Solid Edge part; units mm, degrees
sketch "Sketch1" plane through (0, 0, 0) normal (1, 0, 0) x (0, 1, 0)
  line L0 (-22.5, 0) -> (22.5, 0)
  line L1 (22.5, 0) -> (22.5, 6)
  line L2 (22.5, 6) -> (13.5, 6)
  line L3 (13.5, 6) -> (11, 21)
  arc A0 (-11, 21) -> (11, 21) centre (0, 21) cw
  line L4 (-13.5, 6) -> (-11, 21)
  line L5 (-22.5, 6) -> (-13.5, 6)
  line L6 (-22.5, 0) -> (-22.5, 6)
  dimension "D1" = 22.5
  dimension "D2" = 22.5
  dimension "D3" = 22.5
extrude "Protrusion1" add sketch "Sketch1" along normal mid plane 8
hole "Hole_1" at (0, -18, 6) direction (0, 0, -1) diameter 4.5 end up to next start chamfer 0.4 start chamfer angle 30
hole "Hole1" at (0, 18, 6) direction (0, 0, -1) diameter 4.5 end up to next start chamfer 0.4 start chamfer angle 30
chamfer "Chamfer_1" distance 2 angle 45 4 edges at (4, -22.5, 3) (-4, -22.5, 3) (-4, 22.5, 3) (4, 22.5, 3)
hole "Hole_3" at (4, 0, 21) direction (-1, 0, 0) diameter 12.6 end up to next start chamfer 1 start chamfer angle 30 end chamfer 1 end chamfer angle 30
properties material "Polyethylene, low density"
The model under review builds one solid part; all positions refer to its coordinate system, in mm. A direction names the side the tool comes from. Round coordinates to 2 decimals unless told otherwise and drop trailing zeros. Order: outer loops, then holes, each group sorted by start corner. A loop starts at its lowest first (then second) coordinate and runs counter-clockwise, first axis right, second up. Notation, with made-up numbers: (30, 13) -> (47, 13) arc R4 ccw to (47, 18) -> close; hole circle Ø11 at (13.5, 49.5). An arc over 180 degrees is marked (long way). One line per item, written item: value. Start each with the question number.
Q1. Take a section at B-B (y = -18). Write out the cut boundary in (x, z).
Q2. Take a section at D-D (x = 1). Count the separate pieces of the cut face and the enclosed holes in it, and give its area (3 significant figures).
Q3. Wall thickness on line 1 (Y direction, x = 0, z = 1.1); line 2 (X direction, y = -18, z = 1); line 3 (Y direction, x = 0.05, z = 21): over which ranges is each line inside the solid? List them lowest first.
Q4. Machinability: for faces 5 (the face through (-2, -16, 6)), 6 (the face through (0, 0, 0)), which of the approach directions +Z, -Z, +X, -X, +Y, -Y give a long, thin tool a straight path to every point of the face, cutting with its end or side? Answer none if there is none.
Q5. Clearance check with flat-ended pins moving along their axes: pin 1 Ø1 at (x, y) = (3, -2) entering from +Z; pin 2 Ø4 at (x, z) = (2.5, 17) entering from -Y; pin 3 Ø3 at (x, z) = (-3, 16.5) entering from +Y. State where each tip first meets the part, or that it passes through.
Q6. Take a section at A-A (z = 4). Write out the cut boundary in (x, y).
Q7. Take a section at C-C (x = 3.25). Write out the cut boundary in (y, z), and give its area (3 significant figures).
Q8. Mouldability with a two-part tool opening along Y and no side actions: class faces 1 (the face through (0, -22.5, 3)), 2 (the face through (-2, 16, 6)), 3 (the face through (0.676, 15.854, 2.691)), 4 (the face through (0.676, -20.146, 2.691)) as released by +Y, released by -Y, zero draft, split by the parting line, or undercut.
Reported:
1. outline: (-4, 0) -> (-2.25, 0) -> (-2.25, 5.31) -> (-2.65, 6) -> (-4, 6) -> close; (2.25, 0) -> (4, 0) -> (4, 6) -> (2.65, 6) -> (2.25, 5.31) -> close
2. separate pieces: 3
2. enclosed holes: 1
2. area: 654 mm2
3. line 1: y = -22.5 to -20.25, -15.75 to 15.75, 20.25 to 22.5
3. line 2: x = -4 to -2.25, 2.25 to 4
3. line 3: y = -11 to -6.3, 6.3 to 11
4. face 5: +Z, +X, -X, -Y
4. face 6: -Z, +X, -X, +Y, -Y
5. pin 1: stops at z = 31.9
5. pin 2: stops at y = -12
5. pin 3: stops at y = 12
6. outline: (-4, -20.5) -> (-2, -22.5) -> (2, -22.5) -> (4, -20.5) -> (4, 20.5) -> (2, 22.5) -> (-2, 22.5) -> (-4, 20.5) -> close; hole circle Ø4.5 at (0, -18); hole circle Ø4.5 at (0, 18)
7. outline: (-21.25, 0) -> (21.25, 0) -> (21.25, 6) -> (13.5, 6) -> (11, 21) arc R11 ccw to (-11, 21) -> (-13.5, 6) -> (-21.25, 6) -> close; hole circle Ø13.73 at (0, 21)
7. area: 664 mm2
8. face 1: released by -Y
8. face 2: zero draft
8. face 3: undercut
8. face 4: undercut
